from build123d import *

# Parameters (mm, degrees)
SKETCH1_W                     = 38.1
SKETCH1_H                     = 38.1
BOSS_EXTRUDE1_DEPTH           = 6.35
TAP_DRILL_FOR_2_64_TAP1_D     = 1.778
TAP_DRILL_FOR_2_64_TAP1_DEPTH = 7.62
TAP_DRILL_FOR_2_64_TAP1_TIP   = 0.53416509
TAP_DRILL_FOR_2_64_TAP2_D     = 1.778
TAP_DRILL_FOR_2_64_TAP2_DEPTH = 7.62
TAP_DRILL_FOR_2_64_TAP2_TIP   = 0.53416509


with BuildPart() as part:
    # Sketch1 → Boss-Extrude1 (new body)
    with BuildSketch(Plane.XY):
        Rectangle(SKETCH1_W, SKETCH1_H)
    extrude(amount=BOSS_EXTRUDE1_DEPTH)

    # Tap Drill for #2-64 Tap1
    with Locations(Plane(origin=(0, -19.05, 0), x_dir=(-1, 0, 0), z_dir=(0, -1, 0))):
        with Locations((-15.24, -2.6029), (15.24, -2.6029)):
            Hole(TAP_DRILL_FOR_2_64_TAP1_D / 2, depth=TAP_DRILL_FOR_2_64_TAP1_DEPTH)
            with Locations((0, 0, -(TAP_DRILL_FOR_2_64_TAP1_DEPTH + TAP_DRILL_FOR_2_64_TAP1_TIP / 2))):  # 118° drill point
                Cone(0, TAP_DRILL_FOR_2_64_TAP1_D / 2, TAP_DRILL_FOR_2_64_TAP1_TIP, mode=Mode.SUBTRACT)

    # Tap Drill for #2-64 Tap2
    with Locations(Plane(origin=(19.05, 0, 0), x_dir=(0, 0, -1), z_dir=(1, 0, 0))):
        with Locations((-3.175, 10.5664), (-3.175, -9.525)):
            Hole(TAP_DRILL_FOR_2_64_TAP2_D / 2, depth=TAP_DRILL_FOR_2_64_TAP2_DEPTH)
            with Locations((0, 0, -(TAP_DRILL_FOR_2_64_TAP2_DEPTH + TAP_DRILL_FOR_2_64_TAP2_TIP / 2))):  # 118° drill point
                Cone(0, TAP_DRILL_FOR_2_64_TAP2_D / 2, TAP_DRILL_FOR_2_64_TAP2_TIP, mode=Mode.SUBTRACT)


solid = part.part
The listing builds one solid part. Answer for the finished solid, in the listing's coordinates (mm). A direction names the side the tool comes from. Give positions to 0.01 mm unless a question says otherwise; leave off trailing zeros. Order: outer loops, then holes, each group sorted by start corner. A loop starts at its lowest first (then second) coordinate and runs counter-clockwise, first axis right, second up. Notation, with made-up numbers: (86, 0) - (122, 0) arc R20 ccw to (122, 11) - close; hole circle Ø10 at (24.5, -5). An arc over 180 degrees is marked (long way). One line per item, written item: value. Start each with the question number.
1) A cutting plane is placed at B-B on x = 17. Give the vertices of the cut face in (y, z) (3 decimals).
2) A cutting plane is placed at A-A on y = -16. Give the vertices of the cut face in (x, z), then the cut area to 3 significant figures.
3) A tool of negligible diameter and unlimited length cuts with its end or side. For faces 4 (the face through (15.187, -10.393, 2.982)), 5 (the face through (19.05, 0, 3)), 6 (the face through (-14.4, -15.2, 2.9)), from which of +Z, -Z, +X, -X, +Y, -Y can it reach the whole face along a straight path? Write none if from no direction.
4) Given pin 1 Ø1.4 at (y, z) = (10.57, 3.18) entering from +X, flat-ended and moving along its own axis, determine where the tip first touches the part or whether it passes through.
5) The mould has two halves that part along X. Classify faces 1 (the face through (-19.05, 0, 3)), 2 (the face through (10.99, -9.66, 3.1)), 3 (the face through (-15.383, -10.989, 2.662)): released by +X, released by -X, zero draft, split by the parting line, or undercut.
6) Find the intervals of material crossed by L1, parallel to Z at x = -15.24, y = -15; L2, parallel to X at y = -13, z = 3.25; L3, parallel to Z at x = -14.5, y = -15, in increasing order.
Answer sheet:
1. outline: (-19.05, 0) - (19.05, 0) - (19.05, 6.35) - (-19.05, 6.35) - close; hole circle Ø1.778 at (-9.525, 3.175); hole circle Ø1.778 at (10.566, 3.175)
2. outline: (-19.05, 0) - (19.05, 0) - (19.05, 6.35) - (-19.05, 6.35) - close; hole circle Ø1.78 at (-15.24, 2.6); hole circle Ø1.78 at (15.24, 2.6)
2. area: 237 mm2
3. face 4: +X
3. face 5: +Z, -Z, +X, +Y, -Y
3. face 6: -Y
4. pin 1: stops at x = 11.32
5. face 1: released by -X
5. face 2: released by +X
5. face 3: undercut
6. L1: z = 0 to 1.71, 3.49 to 6.35
6. L2: x = -19.05 to -15.85, -14.63 to 14.63, 15.85 to 19.05
6. L3: z = 0 to 2.11, 3.1 to 6.35
